```python
from build123d import *

# Parameters (mm, degrees)
SKETCH_1_W          = 8
SKETCH_1_H          = 106
EXTRUDE_1_DEPTH     = 2.95
SKETCH_2_R          = 0.7
CUT_EXTRUDE_1_DEPTH = 107.342383366
SKETCH_2_3_R        = 1
CUT_EXTRUDE_2_DEPTH = 1.5
SKETCH_3_R          = 0.3
CUT_EXTRUDE_3_DEPTH = 107.342383366


with BuildPart() as part:
    # Sketch 1 → Extrude 1 (new body)
    with BuildSketch(Plane(origin=(0, 0, 0), x_dir=(1, 0, 0), z_dir=(0, 1, 0))):
        with Locations((4, -53)):
            Rectangle(SKETCH_1_W, SKETCH_1_H)
    extrude(amount=EXTRUDE_1_DEPTH)

    # Sketch 2 → Cut-Extrude 1 (cut, through all)
    with BuildSketch(Plane(origin=(0, 2.95, 0), x_dir=(1, 0, 0), z_dir=(0, 1, 0))):
        with Locations(Location((4, -8, 0), (0, 0, 270))):
            Circle(SKETCH_2_R)
        with Locations(Location((4, -2, 0), (0, 0, 270))):
            Circle(SKETCH_2_R)
        with Locations(Location((4, -104, 0), (0, 0, 270))):
            Circle(SKETCH_2_R)
        with Locations(Location((4, -98, 0), (0, 0, 270))):
            Circle(SKETCH_2_R)
        with Locations(Location((4, -28, 0), (0, 0, 270))):
            Circle(SKETCH_2_R)
    extrude(amount=-CUT_EXTRUDE_1_DEPTH, mode=Mode.SUBTRACT)

    # Sketch 2_3 → Cut-Extrude 2 (cut)
    with BuildSketch(Plane(origin=(0, 2.95, 0), x_dir=(1, 0, 0), z_dir=(0, 1, 0))):
        with Locations(Location((4, -8, 0), (0, 0, 270))):
            Circle(SKETCH_2_3_R)
        with Locations(Location((4, -2, 0), (0, 0, 270))):
            Circle(SKETCH_2_3_R)
        with Locations(Location((4, -104, 0), (0, 0, 270))):
            Circle(SKETCH_2_3_R)
        with Locations(Location((4, -98, 0), (0, 0, 270))):
            Circle(SKETCH_2_3_R)
        with Locations(Location((4, -28, 0), (0, 0, 270))):
            Circle(SKETCH_2_3_R)
    extrude(amount=-CUT_EXTRUDE_2_DEPTH, mode=Mode.SUBTRACT)

    # Sketch 3 → Cut-Extrude 3 (cut, through all)
    with BuildSketch(Plane(origin=(8, 0, 0), x_dir=(0, 0, -1), z_dir=(1, 0, 0))):
        with Locations((-33, 1.475)):
            Circle(SKETCH_3_R)
        with Locations((-36.8, 1.475)):
            Circle(SKETCH_3_R)
    extrude(amount=-CUT_EXTRUDE_3_DEPTH, mode=Mode.SUBTRACT)


solid = part.part
```
Design review of the part built by this model. Coordinates are the model's own, in mm. A direction names the side the tool comes from. Round coordinates to 2 decimals unless told otherwise and drop trailing zeros. Write each loop counter-clockwise with the first axis right and the second up, starting at its lowest first coordinate (ties: lowest second). Pieces come first, ordered by that corner, then holes.
Item 1: Clearance check with flat-ended pins moving along their axes: pin 1 Ø1.6 at (x, z) = (4, 2) entering from +Y; pin 2 Ø1.2 at (x, z) = (4, 2) entering from -Y (1 decimal). State where each tip first meets the part, or that it passes through.
Item 2: For faces 5 (the flat face through (4, 2.95, 52)), 6 (the cylindrical face through (4, 2, 103)), list the 3-axis set-ups (+Z, -Z, +X, -X, +Y, -Y) from which the entire face can be reached by the end or side of a thin tool; tool diameter is ignored.
Item 3: The part is to be moulded in two halves that separate along X. For faces 1 (the flat face through (4, 1, 0)), 2 (the flat face through (8, 1, 54)), 3 (the cylindrical face through (4, 2, 97)), 4 (the cylindrical face through (4.676, 2.21, 1.263)), say which applies: +X half, -X half, draft (parallel to the pull), parting line (faces both ways), or undercut.
Item 4: We need section A-A on y = 2.5. Write out the cut boundary in (x, z), and give its area (3 significant figures).
Item 5: For probe 1 along Z at (x, y) = (6.5, 1.5); probe 2 along X at (y, z) = (1.9, 8); probe 3 along Y at (x, z) = (5, 33) (3 decimals), list the stretches that pass through material, from the lowest coordinate up.
Returned:
1. pin 1: stops at y = 1.45
1. pin 2: passes through
2. face 5: +Z, -Z, +X, -X, +Y
2. face 6: +Y
3. face 1: draft
3. face 2: +X half
3. face 3: undercut
3. face 4: undercut
4. outline: (0, 0) - (8, 0) - (8, 106) - (0, 106) - close; hole circle Ø2 at (4, 2); hole circle Ø2 at (4, 8); hole circle Ø2 at (4, 28); hole circle Ø2 at (4, 98); hole circle Ø2 at (4, 104)
4. area: 832 mm2
5. probe 1: z = 0 to 32.7, 33.3 to 36.5, 37.1 to 106
5. probe 2: x = 0 to 3, 5 to 8
5. probe 3: y = 0 to 1.175, 1.775 to 2.95
